Here's the drawing with two shaded views (mm, measured from the low corner). I have some questions. A direction names the side the tool comes from. Round coordinates to 2 decimals unless told otherwise and drop trailing zeros. Order: outer loops, then holes, each group sorted by start corner. A loop starts at its lowest first (then second) coordinate and runs counter-clockwise, first axis right, second up. Notation, with made-up numbers: (5.5, 6) -> (56.5, 6) arc R6 cw to (56.5, 16) -> close; hole circle Ø9 at (0, 72.25). An arc over 180 degrees is marked (long way). Answer in a Markdown table with one row per item.
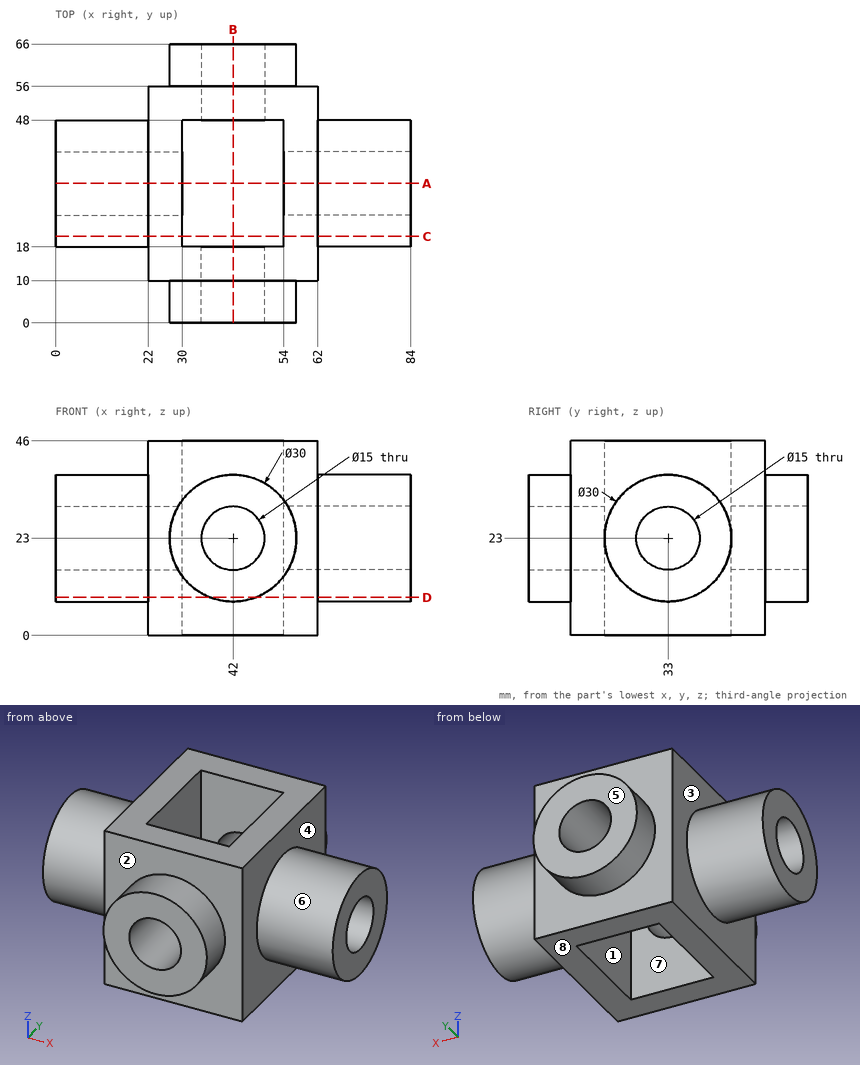
1. Suppose I cut it at A-A on y = 33. Write out the boundary of the cut face in (x, z).
Numbers:
| item | result |
|---|---|
| outline | (0, 8) -> (22, 8) -> (22, 0) -> (30, 0) -> (30, 15.5) -> (0, 15.5) -> close; (0, 30.5) -> (30, 30.5) -> (30, 46) -> (22, 46) -> (22, 38) -> (0, 38) -> close; (54, 0) -> (62, 0) -> (62, 8) -> (84, 8) -> (84, 15.5) -> (54, 15.5) -> close; (54, 30.5) -> (84, 30.5) -> (84, 38) -> (62, 38) -> (62, 46) -> (54, 46) -> close |
2. Suppose I cut it at B-B on x = 42. Write out the boundary of the cut face in (y, z).
Numbers:
| item | result |
|---|---|
| outline | (0, 8) -> (10, 8) -> (10, 0) -> (18, 0) -> (18, 15.5) -> (0, 15.5) -> close; (0, 30.5) -> (18, 30.5) -> (18, 46) -> (10, 46) -> (10, 38) -> (0, 38) -> close; (48, 0) -> (56, 0) -> (56, 8) -> (66, 8) -> (66, 15.5) -> (48, 15.5) -> close; (48, 30.5) -> (66, 30.5) -> (66, 38) -> (56, 38) -> (56, 46) -> (48, 46) -> close |
3. Suppose I cut it at C-C on y = 20.5. Write out the boundary of the cut face in (x, z), then the cut area to 3 significant figures.
Numbers:
| item | result |
|---|---|
| outline | (0, 14.71) -> (22, 14.71) -> (22, 0) -> (30, 0) -> (30, 46) -> (22, 46) -> (22, 31.29) -> (0, 31.29) -> close; (54, 0) -> (62, 0) -> (62, 14.71) -> (84, 14.71) -> (84, 31.29) -> (62, 31.29) -> (62, 46) -> (54, 46) -> close |
| area | 1,470 mm2 |
4. We'd pull the mould along Y, two halves only. Please class the marked faces 5, 6, 7 and 8: released by +Y, released by -Y, zero draft, split by the parting line, or undercut.
Numbers:
| item | result |
|---|---|
| face 5 | released by +Y |
| face 6 | split by the parting line |
| face 7 | undercut |
| face 8 | zero draft |
5. For the marked faces 1, 2, 3 and 4, which set-ups out of +Z, -Z, +X, -X, +Y, -Y let a thin tool reach every point of the face, with its end or its side?
Numbers:
| item | result |
|---|---|
| face 1 | +Z, -Z |
| face 2 | -Y |
| face 3 | -X |
| face 4 | +X |
6. Suppose I cut it at D-D on z = 9. Write out the boundary of the cut face in (x, y), then the cut area to 3 significant figures.
Numbers:
| item | result |
|---|---|
| outline | (0, 27.61) -> (22, 27.61) -> (22, 10) -> (36.61, 10) -> (36.61, 0) -> (47.39, 0) -> (47.39, 10) -> (62, 10) -> (62, 27.61) -> (84, 27.61) -> (84, 38.39) -> (62, 38.39) -> (62, 56) -> (47.39, 56) -> (47.39, 66) -> (36.61, 66) -> (36.61, 56) -> (22, 56) -> (22, 38.39) -> (0, 38.39) -> close; hole (30, 18) -> (54, 18) -> (54, 48) -> (30, 48) -> close |
| area | 1,810 mm2 |
7. For pin 1 Ø4 at (x, z) = (72.5, 32) entering from -Y; pin 2 Ø1 at (y, z) = (13, 14.5) entering from -X; pin 3 Ø24 at (y, z) = (33, 23) entering from -X; pin 4 Ø13.5 at (x, z) = (42, 23) entering from +Y, each with a flat end and sliding along its axis, tell me the tip position at first contact or that it passes through.
Numbers:
| item | result |
|---|---|
| pin 1 | stops at y = 19.73 |
| pin 2 | stops at x = 22 |
| pin 3 | stops at x = 0 |
| pin 4 | passes through |
8. Please list where these lines run through material, in increasing order: line 1 along Y through (x, z) = (31, 6.5); line 2 along X through (y, z) = (27, 43.5); line 3 along X through (y, z) = (21, 24).
Numbers:
| item | result |
|---|---|
| line 1 | y = 10 to 18, 48 to 56 |
| line 2 | x = 22 to 30, 54 to 62 |
| line 3 | x = 0 to 30, 54 to 84 |
